Design review of the part built by this model. Coordinates are the model's own, in mm. A direction names the side the tool comes from. Round coordinates to 2 decimals unless told otherwise and drop trailing zeros. Loops run counter-clockwise (first coordinate to the right, second up) from the corner with the lowest first, then second, coordinate; pieces in that order, holes last. Notation, with made-up numbers: (13.5, 80.5) - (48.5, 80.5) arc R16 ccw to (48.5, 97.5) - close; hole circle Ø9 at (73, 20.5). An arc over 180 degrees is marked (long way). Answer as CSV lines item,"result". Start each with the question number.
(1) Consider section C-C (z = -5). Give the boundary of the cut face in (x, y) (3 decimals), and give its area (3 significant figures).
(2) Consider section B-B (y = 25.4). Give the boundary of the cut face in (x, z) (3 decimals).
(3) For P1, Ø17, axis at y = 25.4, z = 0, coming from the -X side, flat-tipped, find the tip position at first contact; note if it passes through.
(4) Consider section A-A (x = 0). Give the boundary of the cut face in (y, z) (3 decimals).
(5) Consider section D-D (y = 1). Give the boundary of the cut face in (x, z) (3 decimals).
(6) Mouldability with a two-part tool opening along Y and no side actions: class faces 3 (the flat face through (-3, 0, -32)), 4 (the flat face through (0.2, -0.4, -38.1)), 5 (the cylindrical face through (-33.32, 16.1, 2.06)) as released by +Y, released by -Y, zero draft, split by the parting line, or undercut.
(7) For faces 1 (the flat face through (32, -3.175, 9)), 2 (the flat face through (-31.75, 13, 1)), list the 3-axis set-ups (+Z, -Z, +X, -X, +Y, -Y) from which the entire face can be reached by the end or side of a thin tool; tool diameter is ignored.
(8) Wall thickness on L1, parallel to X at y = 2.5, z = 10 (3 decimals); L2, parallel to Y at x = -32.45, z = 0 (3 decimals); L3, parallel to Z at x = -33.55, y = 25.4 (3 decimals): over which ranges is each line inside the solid? List them lowest first.
from build123d import *

# Parameters (mm, degrees)
BOSS_EXTRUDE1_DEPTH = 38.1
SKETCH2_R           = 9.525
CUT_EXTRUDE1_DEPTH  = 70.85
SKETCH3_R           = 31.75
CUT_EXTRUDE2_DEPTH  = 48.625


with BuildPart() as part:
    # Sketch1 → Boss-Extrude1 (new body, symmetric)
    with BuildSketch(Plane.XY):
        Polygon((-31.75, 0), (31.75, 0), (31.75, 44.45), (34.925, 44.45), (34.925, -3.175), (-34.925, -3.175), (-34.925, 44.45), (-31.75, 44.45), align=None)
    extrude(amount=BOSS_EXTRUDE1_DEPTH, both=True)

    # Sketch2 → Cut-Extrude1 (cut, through all)
    with BuildSketch(Plane(origin=(34.925, 0, 0), x_dir=(0, 0, -1), z_dir=(1, 0, 0))):
        with Locations((0, 25.4)):
            Circle(SKETCH2_R)
    extrude(amount=-CUT_EXTRUDE1_DEPTH, mode=Mode.SUBTRACT)

    # Sketch3 → Cut-Extrude2 (cut, through all)
    with BuildSketch(Plane.XZ.offset(3.175)):
        Circle(SKETCH3_R)
    extrude(amount=-CUT_EXTRUDE2_DEPTH, mode=Mode.SUBTRACT)


solid = part.part
Determined:
1,outline,"(-34.925, -3.175) - (-31.354, -3.175) - (-31.354, 0) - (-31.75, 0) - (-31.75, 17.293) - (-34.925, 17.293) - close; (-34.925, 33.507) - (-31.75, 33.507) - (-31.75, 44.45) - (-34.925, 44.45) - close; (31.354, -3.175) - (34.925, -3.175) - (34.925, 17.293) - (31.75, 17.293) - (31.75, 0) - (31.354, 0) - close; (31.75, 33.507) - (34.925, 33.507) - (34.925, 44.45) - (31.75, 44.45) - close"
1,area,"202 mm^2"
2,outline,"(-34.925, -38.1) - (-31.75, -38.1) - (-31.75, -9.525) - (-34.925, -9.525) - close; (-34.925, 9.525) - (-31.75, 9.525) - (-31.75, 38.1) - (-34.925, 38.1) - close; (31.75, -38.1) - (34.925, -38.1) - (34.925, -9.525) - (31.75, -9.525) - close; (31.75, 9.525) - (34.925, 9.525) - (34.925, 38.1) - (31.75, 38.1) - close"
3,P1,"passes through"
4,outline,"(-3.175, -38.1) - (0, -38.1) - (0, -31.75) - (-3.175, -31.75) - close; (-3.175, 31.75) - (0, 31.75) - (0, 38.1) - (-3.175, 38.1) - close"
5,outline,"(-34.925, -38.1) - (-31.75, -38.1) - (-31.75, 38.1) - (-34.925, 38.1) - close; (31.75, -38.1) - (34.925, -38.1) - (34.925, 38.1) - (31.75, 38.1) - close"
6,face 3,"released by +Y"
6,face 4,"zero draft"
6,face 5,"undercut"
7,face 1,"+Z, -Z, +X, -X, -Y"
7,face 2,"+Z, -Z, +Y"
8,L1,"x = -34.925 to -31.75, 31.75 to 34.925"
8,L2,"y = -3.175 to 15.875, 34.925 to 44.45"
8,L3,"z = -38.1 to -9.525, 9.525 to 38.1"
